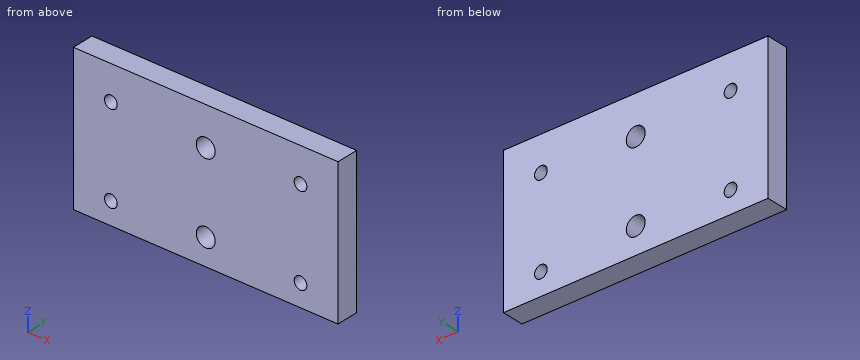
from build123d import *

# Parameters (mm, degrees)
SKETCH1_W               = 76.2
SKETCH1_H               = 152.4
SKETCH1_R               = 2.7305
SKETCH1_R_2             = 1.8288
BOSS_EXTRUDE1_DEPTH     = 6.35
SKETCH2_W               = 76.2
SKETCH2_H               = 110.740191545
CUT_EXTRUDE1_DEPTH      = 1
CUT_EXTRUDE1_DEPTH_BACK = 7.35


with BuildPart() as part:
    # Sketch1 → Boss-Extrude1 (new body)
    with BuildSketch(Plane(origin=(0, 0, 0), x_dir=(1, 0, 0), z_dir=(0, 1, 0))):
        Rectangle(SKETCH1_W, SKETCH1_H)
        with Locations((0, 19.05)):
            Circle(SKETCH1_R, mode=Mode.SUBTRACT)
        with Locations((0, -19.05)):
            Circle(SKETCH1_R, mode=Mode.SUBTRACT)
        with Locations((0, -57.15)):
            Circle(SKETCH1_R, mode=Mode.SUBTRACT)
        with Locations((27.305, 44.45)):
            Circle(SKETCH1_R_2, mode=Mode.SUBTRACT)
        with Locations((27.305, 6.35)):
            Circle(SKETCH1_R_2, mode=Mode.SUBTRACT)
        with Locations((27.305, -31.75)):
            Circle(SKETCH1_R_2, mode=Mode.SUBTRACT)
        with Locations((-27.305, 6.35)):
            Circle(SKETCH1_R_2, mode=Mode.SUBTRACT)
        with Locations((-27.305, -31.75)):
            Circle(SKETCH1_R_2, mode=Mode.SUBTRACT)
        with Locations((-27.305, 44.45)):
            Circle(SKETCH1_R_2, mode=Mode.SUBTRACT)
        with Locations((0, 45.6779905)):
            Circle(SKETCH1_R, mode=Mode.SUBTRACT)
        with Locations((27.305, 69.85)):
            Circle(SKETCH1_R_2, mode=Mode.SUBTRACT)
        with Locations((-27.305, 69.85)):
            Circle(SKETCH1_R_2, mode=Mode.SUBTRACT)
        with Locations((0, 68.6220095)):
            Circle(SKETCH1_R, mode=Mode.SUBTRACT)
    extrude(amount=-BOSS_EXTRUDE1_DEPTH)

    # Sketch2 → Cut-Extrude1 (cut, two sides)
    with BuildSketch(Plane(origin=(0, 0, 0), x_dir=(1, 0, 0), z_dir=(0, 1, 0))) as cut_extrude1_sk:
        with Locations((0, -20.829904228)):
            Rectangle(SKETCH2_W, SKETCH2_H)
    extrude(amount=CUT_EXTRUDE1_DEPTH, mode=Mode.SUBTRACT)
    extrude(cut_extrude1_sk.sketch, amount=-CUT_EXTRUDE1_DEPTH_BACK, mode=Mode.SUBTRACT)


solid = part.part
Build history of the part. All positions in model axes, mm. Round coordinates to 2 decimals unless told otherwise and drop trailing zeros. Loops run counter-clockwise (first coordinate to the right, second up) from the corner with the lowest first, then second, coordinate; pieces in that order, holes last. Notation, with made-up numbers: (-7, 6) -> (6, 6) arc R19 cw to (6, 11) -> close; hole circle Ø4 at (23.25, 33.5). An arc over 180 degrees is marked (long way). One line per item, written item: value. Start each with the question number.
Q1. Probe line 1 along Z through (x, y) = (0, -3.5); line 2 along X through (y, z) = (-3, -45); line 3 along X through (y, z) = (-1.5, -69.85). List the from-to ranges inside material, lowest first.
Q2. Cut at B-B on z = -69.85. List the corners of the cut face in (x, y).
Q3. Cut at A-A on x = 0. List the corners of the cut face in (y, z), plus the area to 3 significant figures.
Q4. Drop a flat-ended pin along its axis: pin 1 Ø3 at (x, z) = (-27.305, -69.85) entering from -Y. Give the stop position or say it passes through.
Q5. Cut at D-D on z = -47.5. List the corners of the cut face in (x, y).
Q6. Cut at C-C on y = -3.25. Count the separate pieces of the cut face and the enclosed holes in it, plus the area to 3 significant figures.
Computed:
1. line 1: -76.2 to -71.35, -65.89 to -48.41, -42.95 to -34.54
1. line 2: -38.1 to -29.05, -25.56 to -2.64, 2.64 to 25.56, 29.05 to 38.1
1. line 3: -38.1 to -29.13, -25.48 to -2.44, 2.44 to 25.48, 29.13 to 38.1
2. outline: (-38.1, -6.35) -> (-29.13, -6.35) -> (-29.13, 0) -> (-38.1, 0) -> close; (-25.48, -6.35) -> (-2.44, -6.35) -> (-2.44, 0) -> (-25.48, 0) -> close; (2.44, -6.35) -> (25.48, -6.35) -> (25.48, 0) -> (2.44, 0) -> close; (29.13, -6.35) -> (38.1, -6.35) -> (38.1, 0) -> (29.13, 0) -> close
3. outline: (-6.35, -76.2) -> (0, -76.2) -> (0, -71.35) -> (-6.35, -71.35) -> close; (-6.35, -65.89) -> (0, -65.89) -> (0, -48.41) -> (-6.35, -48.41) -> close; (-6.35, -42.95) -> (0, -42.95) -> (0, -34.54) -> (-6.35, -34.54) -> close
3. area: 195 mm²
4. pin 1: through
5. outline: (-38.1, -6.35) -> (-2.03, -6.35) -> (-2.03, 0) -> (-38.1, 0) -> close; (2.03, -6.35) -> (38.1, -6.35) -> (38.1, 0) -> (2.03, 0) -> close
6. separate pieces: 1
6. enclosed holes: 6
6. area: 3,090 mm²
